Part model, mm, in its own coordinate system. Face numbers are marked on the shaded views. Coordinates: 2 decimals unless noted, no trailing zeros. Loops run counter-clockwise (first coordinate to the right, second up) from the corner with the lowest first, then second, coordinate; pieces in that order, holes last. Notation, with made-up numbers: M 72,23.5 L 113,23.5 A23 ccw 113,54.5 Z; hole C 27,1.25 d4. An arc over 180 degrees is marked long. Answer as a JSON object with one key per item and string values. Group by question number.
1. Saw through at D-D on x = -49.5. Write the cut outline in (y, z).
2. Drop flat-ended pins along their axis: pin 1 Ø1.5 at (y, z) = (131.5, 488.5) entering from +X; pin 2 Ø8 at (y, z) = (145, 485.5) entering from -X; pin 3 Ø8 at (x, z) = (180.5, 482.5) entering from +Y. Give the stop position or say it passes through.
3. Mould opens along Y. For the marked faces 1, 2 and 3 say: released by +Y, released by -Y, zero draft, split by the parting line, or undercut.
4. Saw through at B-B on y = 150.5. Write the cut outline in (x, z).
5. Drill centre lines: L1, parallel to Y at x = 291, z = 500; L2, parallel to Z at x = 279, y = 128; L3, parallel to Z at x = 178, y = 139.5. Where is each one in solid material? Low to high.
6. Saw through at A-A on z = 500. Write the cut outline in (x, y).
7. Saw through at C-C on x = 38. Write the cut outline in (y, z).
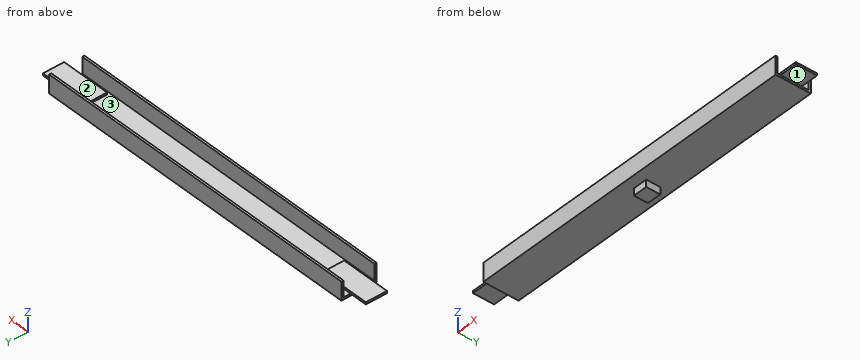
from build123d import *

# Parameters (mm, degrees)
SKETCH1_W           = 477.000009268
SKETCH1_H           = 50.00000447
BOSS_EXTRUDE1_DEPTH = 25.999993086
SKETCH2_W           = 23.000001907
SKETCH2_H           = 43.999992311
CUT_EXTRUDE1_DEPTH  = 722.543490013
SKETCH3_W           = 99.999994039
SKETCH3_H           = 30.000001192
BOSS_EXTRUDE2_DEPTH = 2.999991179
SKETCH4_W           = 99.999995902
SKETCH4_H           = 30.000001192
BOSS_EXTRUDE3_DEPTH = 2.999991179
SKETCH5_W           = 19.999995828
SKETCH5_H           = 19.999995828
BOSS_EXTRUDE4_DEPTH = 10.000020266
MOVE_FACE8_BY       = 30
MOVE_FACE8_2_BY     = 30
MOVE_FACE9_BY       = 5
MOVE_FACE9_2_BY     = 5
MOVE_FACE10_BY      = 5
MOVE_FACE10_2_BY    = 5
MOVE_FACE11_BY      = 2
MOVE_FACE11_2_BY    = 2
MOVE_FACE12_BY      = 2
MOVE_FACE12_2_BY    = 2


with BuildPart() as part:
    # Sketch1 → Boss-Extrude1 (new body)
    with BuildSketch(Plane.XY.offset(513.999998569)):
        with Locations((177.500003949, 144.999999553)):
            Rectangle(SKETCH1_W, SKETCH1_H)
    extrude(amount=-BOSS_EXTRUDE1_DEPTH)

    # Sketch2 → Cut-Extrude1 (cut, through all)
    with BuildSketch(Plane.ZY.offset(61.000000685)):
        with Locations((502.499997616, 144.999999553)):
            Rectangle(SKETCH2_W, SKETCH2_H)
    extrude(amount=-CUT_EXTRUDE1_DEPTH, mode=Mode.SUBTRACT)

    # Sketch3 → Boss-Extrude2 (add)
    with BuildSketch(Plane.XY.offset(490.999996662)):
        with Locations((420.999988914, 144.999995828)):
            Rectangle(SKETCH3_W, SKETCH3_H)
    extrude(amount=BOSS_EXTRUDE2_DEPTH)

    # Sketch4 → Boss-Extrude3 (add)
    with BuildSketch(Plane.XY.offset(490.999996662)):
        with Locations((-65.999998711, 144.999995828)):
            Rectangle(SKETCH4_W, SKETCH4_H)
    extrude(amount=BOSS_EXTRUDE3_DEPTH)

    # Sketch5 → Boss-Extrude4 (add)
    with BuildSketch(Plane(origin=(0, 0, 488.000005484), x_dir=(-1, 0, 0), z_dir=(0, 0, -1))):
        with Locations((-177.500002086, 145.000003278)):
            Rectangle(SKETCH5_W, SKETCH5_H)
    extrude(amount=BOSS_EXTRUDE4_DEPTH)

    # Move Face8: a face moved inward by 30.0
    extrude(part.faces().sort_by_distance((-115.999996662, 144.999995828, 492.499992251))[0], amount=MOVE_FACE8_BY, dir=(1, 0, 0), mode=Mode.SUBTRACT)

    # Move Face8 2: a face moved inward by 30.0
    extrude(part.faces().sort_by_distance((470.999985933, 144.999995828, 492.499992251))[0], amount=MOVE_FACE8_2_BY, dir=(-1, 0, 0), mode=Mode.SUBTRACT)

    # Move Face9: a face moved outward by 5.0
    extrude(part.faces().sort_by_distance((405.999988914, 129.999995232, 492.499992251))[0], amount=MOVE_FACE9_BY, dir=(0, -1, 0))

    # Move Face9 2: a face moved outward by 5.0
    extrude(part.faces().sort_by_distance((-50.999998711, 129.999995232, 492.499992251))[0], amount=MOVE_FACE9_2_BY, dir=(0, -1, 0))

    # Move Face10: a face moved inward by 5.0
    extrude(part.faces().sort_by_distance((-50.999998711, 159.999996424, 492.499992251))[0], amount=MOVE_FACE10_BY, dir=(0, -1, 0), mode=Mode.SUBTRACT)

    # Move Face10 2: a face moved inward by 5.0
    extrude(part.faces().sort_by_distance((405.999988914, 159.999996424, 492.499992251))[0], amount=MOVE_FACE10_2_BY, dir=(0, -1, 0), mode=Mode.SUBTRACT)

    # Move Face11: a face moved outward by 2.0
    extrude(part.faces().sort_by_distance((-50.999998711, 154.999996424, 492.499992251))[0], amount=MOVE_FACE11_BY, dir=(0, 1, 0))

    # Move Face11 2: a face moved outward by 2.0
    extrude(part.faces().sort_by_distance((405.999988914, 154.999996424, 492.499992251))[0], amount=MOVE_FACE11_2_BY, dir=(0, 1, 0))

    # Move Face12: a face moved inward by 2.0
    extrude(part.faces().sort_by_distance((405.999988914, 124.999995232, 492.499992251))[0], amount=MOVE_FACE12_BY, dir=(0, 1, 0), mode=Mode.SUBTRACT)

    # Move Face12 2: a face moved inward by 2.0
    extrude(part.faces().sort_by_distance((-50.999998711, 124.999995232, 492.499992251))[0], amount=MOVE_FACE12_2_BY, dir=(0, 1, 0), mode=Mode.SUBTRACT)


solid = part.part
Outcome:
{
 "1": {"outline": "M 120,488 L 170,488 L 170,514 L 167,514 L 167,491 L 157,491 L 157,494 L 127,494 L 127,491 L 123,491 L 123,514 L 120,514 Z"},
 "2": {"pin 1": "stops at x = 416", "pin 2": "stops at x = -61", "pin 3": "stops at y = 155"},
 "3": {"face 1": "zero draft", "face 2": "undercut", "face 3": "undercut"},
 "4": {"outline": "M -86,491 L -61,491 L -61,488 L 167.5,488 L 167.5,478 L 187.5,478 L 187.5,488 L 416,488 L 416,491 L 441,491 L 441,494 L 371,494 L 371,491 L -16,491 L -16,494 L -86,494 Z"},
 "5": {"L1": "y = 120 to 123, 167 to 170", "L2": "z = 488 to 491", "L3": "z = 478 to 491"},
 "6": {"outline": "M -61,120 L 416,120 L 416,123 L -61,123 Z; M -61,167 L 416,167 L 416,170 L -61,170 Z"},
 "7": {"outline": "M 120,488 L 170,488 L 170,514 L 167,514 L 167,491 L 123,491 L 123,514 L 120,514 Z"}
}
